```python
from build123d import *

# Parameters (mm, degrees)
BOSS_EXTRUDE1_REACH = 164.942
CUT_EXTRUDE1_DEPTH  = 163.941707368


with BuildPart() as part:
    # Sketch1 → Revolve1 (revolve)
    with BuildSketch(Plane.XY, mode=Mode.PRIVATE) as revolve1_sk:
        Polygon((-78.541169384, 30), (71.458830616, 45), (71.458830616, 39.975062189), (-78.541169384, 24.975062189), align=None)
    revolve(revolve1_sk.sketch.rotate(Axis((-78.541169384, 0, 0), (1, 0, 0)), 90), axis=Axis((-78.541169384, 0, 0), (1, 0, 0)))

    # Sketch3 → Boss-Extrude1 (add, up to next)
    with BuildSketch(Plane(origin=(71.458830616, 0, 0), x_dir=(0, 0, -1), z_dir=(1, 0, 0)), mode=Mode.PRIVATE) as boss_extrude1_sk1:
        with BuildLine():
            Line((-20.615528128, -40), (20.615528128, -40))
            ThreePointArc((20.615528128, -40), (24.577379737, -37.69552235), (28.284271247, -35))
            Line((28.284271247, -35), (-28.284271247, -35))
            ThreePointArc((-28.284271247, -35), (-24.577379737, -37.69552235), (-20.615528128, -40))
        make_face()
    boss_extrude1_tool1 = extrude(boss_extrude1_sk1.sketch, amount=-BOSS_EXTRUDE1_REACH, mode=Mode.PRIVATE) - part.part
    add(boss_extrude1_tool1.solids().sort_by_distance((71.458831, -37.37172, 0))[0])

    # Sketch4 → Cut-Extrude1 (cut, through all)
    with BuildSketch(Plane(origin=(71.458830616, 0, 0), x_dir=(0, 0, -1), z_dir=(1, 0, 0))):
        with BuildLine():
            Line((-20.615528128, -40), (20.615528128, -40))
            ThreePointArc((20.615528128, -40), (0, -45), (-20.615528128, -40))
        make_face()
    extrude(amount=-CUT_EXTRUDE1_DEPTH, mode=Mode.SUBTRACT)


solid = part.part
```
CAD build for the part. Positions are in the model's coordinates, mm. Round coordinates to 2 decimals unless told otherwise and drop trailing zeros. Write each loop counter-clockwise with the first axis right and the second up, starting at its lowest first coordinate (ties: lowest second). Pieces come first, ordered by that corner, then holes. Notation, with made-up numbers: (55.5, 56.25) - (99.5, 56.25) arc R25 cw to (99.5, 93.25) - close; hole circle Ø4 at (43, 64.25). An arc over 180 degrees is marked (long way). Return JSON: item names as keys, results as strings. Group by question number.
Item 1: Band-saw the part on C-C on x = 3. List the corners of the cut face in (y, z).
Item 2: Probe probe 1 along Z at (x, y) = (-4.5, 8.5); probe 2 along Z at (x, y) = (-52, 21); probe 3 along Y at (x, z) = (-53, 15). List the from-to ranges inside material, lowest first.
Item 3: Band-saw the part on A-A on y = 0. List the corners of the cut face in (x, z), plus the area to 3 significant figures.
Item 4: Mould opens along Y. For faces 1 (the face through (52, -35, 0)), 2 (the face through (52, -40, 0)), 3 (the face through (-2.5, 36.7, -8.2)), 4 (the face through (-4.59, 31.6, -7.02)) say: +Y half, -Y half, draft (parallel to the pull), parting line (faces both ways), or undercut.
Item 5: Band-saw the part on B-B on x = 27. List the corners of the cut face in (y, z), plus the area to 3 significant figures.
Item 6: Band-saw the part on D-D on x = -28. List the corners of the cut face in (y, z), plus the area to 3 significant figures.
Item 7: Flat gauge pins, fed straight in: pin 1 Ø3 at (y, z) = (-6, -22.5) entering from +X; pin 2 Ø4 at (x, z) = (35.5, -17) entering from +Y; pin 3 Ø8 at (x, z) = (-40, 34) entering from -Y; pin 4 Ø12 at (x, y) = (-19, -11) entering from +Z. Where does each tip first touch, or does it go through?
Resolved:
{
 "1": {"outline": "circle Ø76.31 at (0, 0); hole circle Ø66.26 at (0, 0)"},
 "2": {"probe 1": "z = -36.43 to -31.24, 31.24 to 36.43", "probe 2": "z = -25.01 to -17.95, 17.95 to 25.01", "probe 3": "y = -28.89 to -23.08, 23.08 to 28.89"},
 "3": {"outline": "(-78.54, -30) - (71.46, -45) - (71.46, -39.98) - (-78.54, -24.98) - close; (-78.54, 24.98) - (71.46, 39.98) - (71.46, 45) - (-78.54, 30) - close", "area": "1,510 mm²"},
 "4": {"face 1": "undercut", "face 2": "-Y half", "face 3": "parting line", "face 4": "undercut"},
 "5": {"outline": "(-40, -6.68) arc R40.55 ccw (long way) to (-40, 6.68) - close; hole (-35, -6.11) arc R35.53 ccw (long way) to (-35, 6.11) - close", "area": "1,200 mm²"},
 "6": {"outline": "circle Ø70.11 at (0, 0); hole circle Ø60.06 at (0, 0)", "area": "1,030 mm²"},
 "7": {"pin 1": "passes through", "pin 2": "stops at y = 38.62", "pin 3": "stops at y = -15.74", "pin 4": "stops at z = 35.79"}
}
